Could you check a few things on this model? Use its own coordinates, in mm. Give positions to 0.01 mm unless a question says otherwise; leave off trailing zeros. Loops run counter-clockwise (first coordinate to the right, second up) from the corner with the lowest first, then second, coordinate; pieces in that order, holes last. Notation, with made-up numbers: M -15,45.25 L 33,45.25 A19 ccw 33,51.25 Z; hole C 50.5,-20 d4. An arc over 180 degrees is marked long. Return JSON: item names as keys, results as strings. Group by question number.
1. If we section it at B-B (x = 84): Write out the boundary of the cut face in (y, z).
2. If we section it at A-A (y = 3.9): State how many separate pieces and enclosed holes the cut face has, plus the area to 3 significant figures.
3. For pin 1 (2.5 mm diameter, centred on x = 0, z = -130, fed in from -Y); pin 2 (1 mm diameter, centred on y = 2, z = 72, fed in from -X); pin 3 (1.5 mm diameter, centred on y = 3, z = 77.5, fed in from -X); pin 4 (2.5 mm diameter, centred on x = -59, y = 2.5, fed in from +Z), each with a flat end and sliding along its axis, tell me the tip position at first contact or that it passes through.
4. Please list where these lines run through material, in increasing order: line 1 (Z direction, x = -99, y = 2.7); line 2 (X direction, y = 3.6, z = 17.5); line 3 (X direction, y = 3.6, z = -21.5).
5. If we section it at C-C (z = -48): Write out the boundary of the cut face in (x, y), plus the area to 3 significant figures.
```python
from build123d import *

# Parameters (mm, degrees)
SKETCH1_R           = 150
BOSS_EXTRUDE1_DEPTH = 5
SKETCH2_R           = 1.5
CUT_EXTRUDE1_DEPTH  = 5
SKETCH3_R           = 1.5
CUT_EXTRUDE2_DEPTH  = 5
SKETCH4_R           = 1.5
CUT_EXTRUDE3_DEPTH  = 5
SKETCH5_R           = 1.5
SKETCH5_W           = 20
SKETCH5_H           = 20
CUT_EXTRUDE4_DEPTH  = 5
SKETCH6_R           = 1.25
CUT_EXTRUDE5_DEPTH  = 5


with BuildPart() as part:
    # Sketch1 → Boss-Extrude1 (new body)
    with BuildSketch(Plane(origin=(0, 0, 0), x_dir=(1, 0, 0), z_dir=(0, 1, 0))):
        with Locations(Location((0, 0, 0), (0, 0, 270))):
            Circle(SKETCH1_R)
    extrude(amount=BOSS_EXTRUDE1_DEPTH)

    # Sketch2 → Cut-Extrude1 (cut)
    with BuildSketch(Plane(origin=(0, 5, 0), x_dir=(1, 0, 0), z_dir=(0, 1, 0))):
        with Locations(Location((0, 130, 0), (0, 0, 270))):
            Circle(SKETCH2_R)
        with Locations(Location((112.583302492, 65, 0), (0, 0, 270))):
            Circle(SKETCH2_R)
        with Locations(Location((112.583302492, -65, 0), (0, 0, 270))):
            Circle(SKETCH2_R)
        with Locations(Location((0, -130, 0), (0, 0, 270))):
            Circle(SKETCH2_R)
        with Locations(Location((-112.583302492, -65, 0), (0, 0, 270))):
            Circle(SKETCH2_R)
        with Locations(Location((-112.583302492, 65, 0), (0, 0, 270))):
            Circle(SKETCH2_R)
    extrude(amount=-CUT_EXTRUDE1_DEPTH, mode=Mode.SUBTRACT)

    # Sketch3 → Cut-Extrude2 (cut)
    with BuildSketch(Plane(origin=(0, 5, 0), x_dir=(1, 0, 0), z_dir=(0, 1, 0))):
        with Locations(Location((-10.1, 6.25, 0), (0, 0, 270))):
            Circle(SKETCH3_R)
        with Locations(Location((10.1, 6.25, 0), (0, 0, 270))):
            Circle(SKETCH3_R)
    extrude(amount=-CUT_EXTRUDE2_DEPTH, mode=Mode.SUBTRACT)

    # Sketch4 → Cut-Extrude3 (cut)
    with BuildSketch(Plane(origin=(0, 5, 0), x_dir=(1, 0, 0), z_dir=(0, 1, 0))):
        with Locations(Location((-21.5, 21.5, 0), (0, 0, 270))):
            Circle(SKETCH4_R)
        with Locations(Location((21.5, 21.5, 0), (0, 0, 270))):
            Circle(SKETCH4_R)
        with Locations(Location((-21.5, -21.5, 0), (0, 0, 270))):
            Circle(SKETCH4_R)
        with Locations(Location((21.5, -21.5, 0), (0, 0, 270))):
            Circle(SKETCH4_R)
    extrude(amount=-CUT_EXTRUDE3_DEPTH, mode=Mode.SUBTRACT)

    # Sketch5 → Cut-Extrude4 (cut)
    with BuildSketch(Plane(origin=(0, 5, 0), x_dir=(1, 0, 0), z_dir=(0, 1, 0))):
        with Locations(Location((-30, -97.5, 0), (0, 0, 270))):
            Circle(SKETCH5_R)
        with Locations(Location((-24, -71.5, 0), (0, 0, 270))):
            Circle(SKETCH5_R)
        with Locations(Location((8, -71.5, 0), (0, 0, 270))):
            Circle(SKETCH5_R)
        with Locations((-60, -81.5)):
            Rectangle(SKETCH5_W, SKETCH5_H)
    extrude(amount=-CUT_EXTRUDE4_DEPTH, mode=Mode.SUBTRACT)

    # Sketch6 → Cut-Extrude5 (cut)
    with BuildSketch(Plane(origin=(0, 5, 0), x_dir=(1, 0, 0), z_dir=(0, 1, 0))):
        with Locations(Location((-50, 40.5, 0), (0, 0, 270))):
            Circle(SKETCH6_R)
        with Locations(Location((-99, 40.5, 0), (0, 0, 270))):
            Circle(SKETCH6_R)
        with Locations(Location((-99, -17.5, 0), (0, 0, 270))):
            Circle(SKETCH6_R)
        with Locations(Location((-50, -17.5, 0), (0, 0, 270))):
            Circle(SKETCH6_R)
    extrude(amount=-CUT_EXTRUDE5_DEPTH, mode=Mode.SUBTRACT)


solid = part.part
```
Answer:
{
 "1": {"outline": "M 0,-124.27 L 5,-124.27 L 5,124.27 L 0,124.27 Z"},
 "2": {"separate pieces": "1", "enclosed holes": "20", "area": "70,200 mm²"},
 "3": {"pin 1": "passes through", "pin 2": "stops at x = -131.86", "pin 3": "stops at x = -128.88", "pin 4": "stops at z = 138.44"},
 "4": {"line 1": "z = -112.69 to -41.75, -39.25 to 16.25, 18.75 to 112.69", "line 2": "x = -148.98 to -100.25, -97.75 to -51.25, -48.75 to 148.98", "line 3": "x = -148.45 to -23, -20 to 20, 23 to 148.45"},
 "5": {"outline": "M -142.11,0 L 142.11,0 L 142.11,5 L -142.11,5 Z", "area": "1,420 mm²"}
}
